For this review, take the finished solid that the model builds, in its own axes (mm). Face numbers are marked on the shaded views. A direction names the side the tool comes from. Round coordinates to 2 decimals unless told otherwise and drop trailing zeros. Loops run counter-clockwise (first coordinate to the right, second up) from the corner with the lowest first, then second, coordinate; pieces in that order, holes last.
1) Take a section at A-A (z = -4.5). State the section outline as (x, y) points, then the cut area to 3 significant figures.
2) Insertion check: pin 1 (3 mm diameter, centred on x = -0.5, z = -6, fed in from +Y); pin 2 (1 mm diameter, centred on y = 1, z = -5.5, fed in from +X); pin 3 (1 mm diameter, centred on x = 0, y = -0.5, fed in from +Z). Each pin has a flat end and moves straight along its axis. Give the tip position at first contact, or say it passes through.
3) Take a section at B-B (z = -1.5). State the section outline as (x, y) points, then the cut area to 3 significant figures.
4) Wall thickness on L1, parallel to X at y = 0.25, z = -1; L2, parallel to X at y = 0, z = -2; L3, parallel to Y at x = -0.25, z = -7: over which ranges is each line inside the solid? List them lowest first.
5) Mouldability with a two-part tool opening along X and no side actions: class the marked faces 1, 2 and 3 as pulls with the +X half, pulls with the -X half, needs draft (parallel to the pull), parting line crosses it, or undercut.
6) Tool access review of the marked faces 4 and 5: name each direction out of +Z, -Z, +X, -X, +Y, -Y from which nothing blocks a thin tool from reaching the whole face with its end or side.
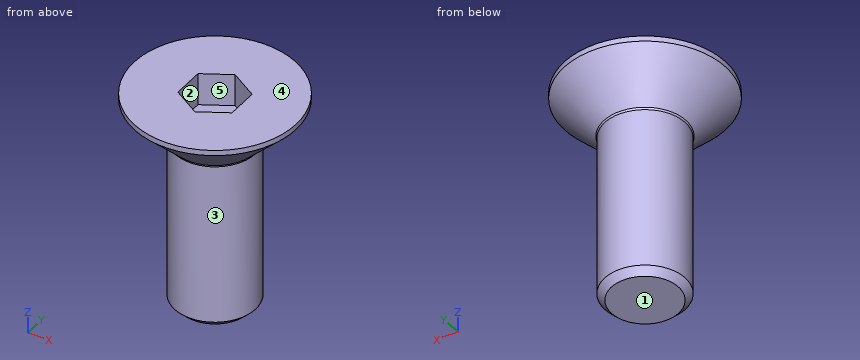
Autodesk Inventor part; units mm, degrees
ref_plane "MSC_PF1" through (0, 0, 0) normal (1, 0, 0) x (0, 1, 0)
ref_plane "MSC_PT1" through (0, 0, 0) normal (0, 0, -1) x (-1, 0, 0)
ref_plane "YZ Plane" through (0, 0, 0) normal (1, 0, 0) x (0, 1, 0)
sketch "Sketch1" plane through (0, 0, 0) normal (0, 1, 0) x (-1, 0, 0)
  point P0 (0, 0)
sketch "Sketch2" plane through (0, 0, 0) normal (0, 1, 0) x (-1, 0, 0)
  line L0 (-1.5, -8) -> (0, -8)
  line L1 (-1.5, -1.7) -> (-1.5, -8)
  line L2 (-3, -0.2) -> (-1.5, -1.7)
  line L3 (-3, 0) -> (-3, -0.2)
  line L4 (0, 0) -> (-3, 0)
  line L5 (0, -8) -> (0, 0)
  line L6 (0, -8) -> (0, 0)
  line L7 (0, -9.6) -> (0, 1.6)
  line L8 (0.6, 0) -> (-3.6, 0)
  dimension "d3" = 3
  dimension "d5" = 1.5
  dimension "d7" = 8
  dimension "ParC" = 0.2
  dimension "d22" = 0
  dimension "d23" = 0
  dimension "d43" = 45
revolve "Revolution1" add sketch "Sketch2" angle 360 about axis through (0, 0, -8) along (0, 0, -1)
sketch "Sketch3" plane through (0, 0, 0) normal (0, 0, 1) x (1, 0, 0)
  line L0 (-1, 0.5774) -> (-1, -0.5774)
  line L1 (0, 1.1547) -> (-1, 0.5774)
  line L2 (1, 0.5774) -> (0, 1.1547)
  line L3 (1, -0.5774) -> (1, 0.5774)
  line L4 (0, -1.1547) -> (1, -0.5774)
  line L5 (-1, -0.5774) -> (0, -1.1547)
  circle A0 centre (0, 0) radius 1 construction
  circle A1 centre (0, 0) radius 1.5 construction
  dimension "d11" = 2
  dimension "d13" = 120
  dimension "d15" = 120
extrude "Extrusion1" cut sketch "Sketch3" against normal blind 1.2
fillet "Fillet1" radius 0.1 1 edges at (-1.5, 0, -1.7)
chamfer "Chamfer1" distance 0.25 angle 45 1 edges at (-1.5, 0, -8) measured on face at (1.4041, 0.5277, -5.9138)
thread "Thread1"
ref_plane "MSC_PF1" through (0, 0, 0) normal (1, 0, 0) x (0, 1, 0)
ref_plane "MSC_PT1" through (0, 0, 0) normal (0, 0, -1) x (-1, 0, 0)
equation "\"d3\" = 0.5 * dk"
equation "\"d5\" = 0.5 * NND"
equation "\"d7\" = NLG"
equation "\"d43\" = 0.5 * ang"
equation "\"d18\" = r"
equation "\"d19\" = 0.5 * PTC"
equation "\"d39\" = 0.5 * PTC"
equation "\"d11\" = ParS"
equation "\"d16\" = ParT"
equation "\"NND\" = 3"
equation "\"PTC\" = 0.5"
equation "\"dk\" = 6"
equation "\"ParK\" = 1.7"
equation "\"ParS\" = 2"
equation "\"ParT\" = 1.2"
equation "\"r\" = 0.1"
equation "\"NLG\" = 8"
equation "\"ang\" = 90deg"
equation "\"THREADDIA\" = NND"
properties part number "CSK Allen Key 3x8mm" material "Steel, Mild"
Response:
1. outline: circle Ø3 at (0, 0)
1. area: 7.07 mm2
2. pin 1: stops at y = 1.5
2. pin 2: stops at x = 1.41
2. pin 3: stops at z = -1.2
3. outline: circle Ø3.4 at (0, 0)
3. area: 9.08 mm2
4. L1: x = -2.19 to -1, 1 to 2.19
4. L2: x = -1.5 to 1.5
4. L3: y = -1.48 to 1.48
5. face 1: needs draft
5. face 2: undercut
5. face 3: parting line crosses it
6. face 4: +Z, +X, -X, +Y, -Y
6. face 5: +Z
